from build123d import *

# Parameters (mm, degrees)
SKETCH1_R           = 13.2
SKETCH1_R_2         = 6
BOSS_EXTRUDE1_DEPTH = 6
CUT_EXTRUDE1_DEPTH  = 2.54
SKETCH3_R           = 13.2
SKETCH3_R_2         = 6
BOSS_EXTRUDE2_DEPTH = 6


with BuildPart() as part:
    # Sketch1 → Boss-Extrude1 (new body)
    with BuildSketch(Plane.XY):
        Circle(SKETCH1_R)
        Circle(SKETCH1_R_2, mode=Mode.SUBTRACT)
    extrude(amount=BOSS_EXTRUDE1_DEPTH)

    # Sketch2 → Cut-Extrude1 (cut)
    with BuildSketch(Plane.XY.offset(6)):
        with BuildLine():
            ThreePointArc((-2.819851171, 12.895287487), (0, 13.2), (2.819851171, 12.895287487))
            ThreePointArc((2.819851171, 12.895287487), (1.826256171, 11.910750525), (1.819851171, 10.512))
            ThreePointArc((1.819851171, 10.512), (0, 10.668364555), (-1.819851171, 10.512))
            ThreePointArc((-1.819851171, 10.512), (-1.826256171, 11.910750525), (-2.819851171, 12.895287487))
        make_face()
    extrude(amount=-CUT_EXTRUDE1_DEPTH, mode=Mode.SUBTRACT)

    # Sketch3 → Boss-Extrude2 (add)
    with BuildSketch(Plane.XY):
        Circle(SKETCH3_R)
        Circle(SKETCH3_R_2, mode=Mode.SUBTRACT)
    extrude(amount=BOSS_EXTRUDE2_DEPTH)


solid = part.part
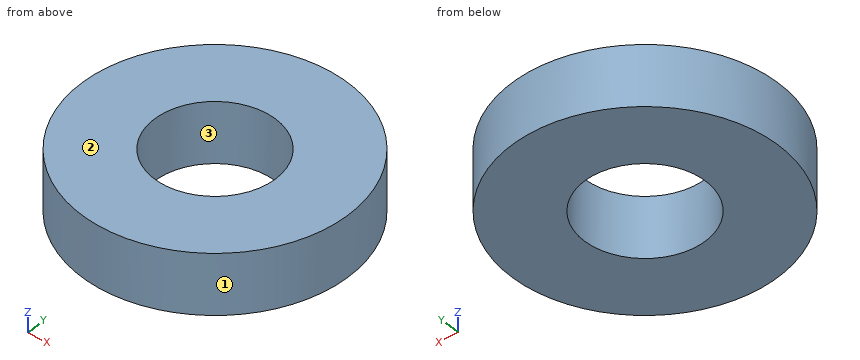
Input: part model. Units: mm. Frame: model coordinates. Face numbers are marked on the shaded views. Coordinates: 2 decimals unless noted, no trailing zeros. Loops run counter-clockwise (first coordinate to the right, second up) from the corner with the lowest first, then second, coordinate; pieces in that order, holes last.
(1) Pull-direction query (X, two-part tool) for the marked faces 1, 2 and 3; classes: released by +X, released by -X, zero draft, split by the parting line, or undercut.
(2) First-contact query: pin 1 Ø7 at (x, y) = (0, 0) entering from -Z (3 decimals); pin 2 Ø3 at (y, z) = (-4.5, 4) entering from +X; pin 3 Ø1 at (y, z) = (-4, 1) entering from +X. Flat tips, straight axial feed; report the tip coordinate or a pass-through.
(3) Section A-A on y = 0. Return the cut outline in (x, z).
(4) Section C-C on z = 4.05. Return the cut outline in (x, y), then the cut area to 3 significant figures.
(5) Material intervals for probe 1 along Y at (x, z) = (0, 1.35); probe 2 along Y at (x, z) = (-5, 4.95); probe 3 along X at (y, z) = (-1.25, 2.35), sorted ascending.
(6) Section D-D on y = -7. Return the cut outline in (x, z).
Data:
1. face 1: split by the parting line
1. face 2: zero draft
1. face 3: undercut
2. pin 1: passes through
2. pin 2: stops at x = 12.85
2. pin 3: stops at x = 12.73
3. outline: (-13.2, 0) - (-6, 0) - (-6, 6) - (-13.2, 6) - close; (6, 0) - (13.2, 0) - (13.2, 6) - (6, 6) - close
4. outline: circle Ø26.4 at (0, 0); hole circle Ø12 at (0, 0)
4. area: 434 mm2
5. probe 1: y = -13.2 to -6, 6 to 13.2
5. probe 2: y = -12.22 to -3.32, 3.32 to 12.22
5. probe 3: x = -13.14 to -5.87, 5.87 to 13.14
6. outline: (-11.19, 0) - (11.19, 0) - (11.19, 6) - (-11.19, 6) - close
